from build123d import *

# Parameters (mm, degrees)
SKETCH1_R           = 13
BOSS_EXTRUDE1_DEPTH = 1
CUT_EXTRUDE1_DEPTH  = 1


with BuildPart() as part:
    # Sketch1 → Boss-Extrude1 (new body)
    with BuildSketch(Plane(origin=(0, 0, 0), x_dir=(1, 0, 0), z_dir=(0, 1, 0))):
        with Locations(Location((0, 0, 0), (0, 0, 270))):
            Circle(SKETCH1_R)
    extrude(amount=BOSS_EXTRUDE1_DEPTH)

    # Sketch2 → Cut-Extrude1 (cut)
    with BuildSketch(Plane(origin=(0, 1, 0), x_dir=(1, 0, 0), z_dir=(0, 1, 0))):
        with BuildLine():
            Line((5.25239325, -1.5848325), (7.730691862, -2.231533889))
            add(Edge.make_bspline(
                [(7.730691862, -2.231533889), (7.745854907, -2.465826289), (7.774011213, -2.900884585), (7.780007907, -3.336797312), (7.782775195, -3.5379575)],
                knots=[0, 0, 0, 0, 1.077062099, 2, 2, 2, 2], degree=3))
            add(Edge.make_bspline(
                [(7.782775195, -3.5379575), (7.775734441, -3.772666286), (7.76198387, -4.231051786), (7.665106789, -4.902107863), (7.503534805, -5.53719048), (7.262506376, -6.13254792), (6.970171749, -6.697349561), (6.599918526, -7.220612544), (6.167294917, -7.709069047), (5.673484979, -8.159929958), (5.121589843, -8.561266158), (4.525330961, -8.915315997), (3.88158819, -9.210662332), (3.194771896, -9.454210567), (2.461957382, -9.639228793), (1.685716726, -9.772679799), (0.864809488, -9.857517539), (0.301796476, -9.866054195), (0.013677973, -9.870422778)],
                knots=[0, 0, 0, 0, 0.99838358, 1.9498399, 2.87846334, 3.779167422, 4.676774372, 5.578403417, 6.498521769, 7.448363946, 8.417281084, 9.396931457, 10.393890904, 11.425717394, 12.493153504, 13.605299621, 14.774526564, 16, 16, 16, 16], degree=3))
            add(Edge.make_bspline(
                [(0.013677973, -9.870422778), (-0.345453387, -9.863405493), (-1.042591343, -9.849783693), (-2.054913482, -9.730806098), (-2.997808304, -9.537362324), (-3.874251245, -9.270503592), (-4.678201905, -8.917315993), (-5.411628354, -8.48501399), (-6.080262751, -7.979187866), (-6.671165693, -7.386273411), (-7.201957369, -6.724194549), (-7.653742039, -5.97838427), (-8.036288232, -5.157199578), (-8.347723272, -4.258020447), (-8.589436148, -3.28160554), (-8.760231838, -2.227786178), (-8.865609009, -1.096529571), (-8.877670491, -0.316264728), (-8.883891472, 0.086174444)],
                knots=[0, 0, 0, 0, 1.125976169, 2.185720361, 3.191248848, 4.14129961, 5.053465363, 5.93822711, 6.80577772, 7.675236456, 8.556734678, 9.460955445, 10.40277975, 11.392896532, 12.440517575, 13.553427658, 14.738125192, 16, 16, 16, 16], degree=3))
            add(Edge.make_bspline(
                [(-8.883891472, 0.086174444), (-8.877144448, 0.471355807), (-8.86396985, 1.223481467), (-8.739062258, 2.323761593), (-8.537683843, 3.368297285), (-8.25053484, 4.357501558), (-7.88374945, 5.291207721), (-7.443760547, 6.173716613), (-6.907249974, 6.992501414), (-6.303194776, 7.754037533), (-5.634782916, 8.444869562), (-4.903943631, 9.039841274), (-4.13324793, 9.555570007), (-3.305494781, 9.969042017), (-2.430073405, 10.289949015), (-1.506733392, 10.522051081), (-0.534275431, 10.656589456), (0.130450492, 10.675493327), (0.469407139, 10.685132778)],
                knots=[0, 0, 0, 0, 1.163899941, 2.272693063, 3.342163629, 4.375955692, 5.38130337, 6.37089149, 7.350964679, 8.334427181, 9.30546345, 10.250064938, 11.177916844, 12.10296145, 13.039623816, 13.99100338, 14.975573636, 16, 16, 16, 16], degree=3))
            add(Edge.make_bspline(
                [(0.469407139, 10.685132778), (0.731368093, 10.679403838), (1.24032138, 10.668273314), (1.980031414, 10.603376578), (2.666696134, 10.474000255), (3.305409253, 10.309794879), (3.889173706, 10.08444307), (4.428427211, 9.822804709), (4.914586315, 9.502127233), (5.349181396, 9.133633154), (5.732807037, 8.715102812), (6.062391941, 8.247124839), (6.347469876, 7.733536448), (6.571984508, 7.166341162), (6.748453612, 6.552678606), (6.879804132, 5.890982879), (6.951396325, 5.180354064), (6.961564938, 4.691361745), (6.966802973, 4.439473056)],
                knots=[0, 0, 0, 0, 1.216450272, 2.363391781, 3.442411128, 4.457483076, 5.420551553, 6.342768242, 7.235147886, 8.116718114, 8.981990498, 9.863560726, 10.768467107, 11.70271401, 12.689043052, 13.729727606, 14.830542089, 16, 16, 16, 16], degree=3))
            Line((6.966802973, 4.439473056), (4.475483528, 3.302320278))
            add(Edge.make_bspline(
                [(4.475483528, 3.302320278), (4.470106952, 3.438293944), (4.45992788, 3.695722764), (4.461276647, 4.056170034), (4.447142903, 4.368506474), (4.448715354, 4.55954313), (4.449441862, 4.647806389)],
                knots=[0, 0, 0, 0, 1.21319996, 2.296861169, 3.213111309, 4, 4, 4, 4], degree=3))
            add(Edge.make_bspline(
                [(4.449441862, 4.647806389), (4.447722623, 4.824448026), (4.444391201, 5.166731988), (4.396660933, 5.661731695), (4.337462463, 6.125936258), (4.234766253, 6.552649254), (4.115177918, 6.949061221), (3.964373313, 7.308698933), (3.783801492, 7.63357582), (3.580758496, 7.927608424), (3.344642243, 8.184947546), (3.080877209, 8.407247168), (2.794090455, 8.602656301), (2.472644536, 8.751215907), (2.129602996, 8.876345015), (1.755447324, 8.955010862), (1.356440833, 9.009630083), (1.080143634, 9.015466719), (0.938157139, 9.018466111)],
                knots=[0, 0, 0, 0, 1.322247294, 2.562159472, 3.722092324, 4.823306397, 5.844541812, 6.820517713, 7.73713301, 8.62386865, 9.490450857, 10.343654022, 11.203094787, 12.080246692, 12.988369862, 13.932056947, 14.937303798, 16, 16, 16, 16], degree=3))
            add(Edge.make_bspline(
                [(0.938157139, 9.018466111), (0.786942196, 9.012673682), (0.491913679, 9.001372339), (0.064405318, 8.885963451), (-0.332873883, 8.703985183), (-0.69991465, 8.444701136), (-1.036329743, 8.114914494), (-1.33955244, 7.710706144), (-1.612917553, 7.235906282), (-1.860109833, 6.690970947), (-2.074074797, 6.070923113), (-2.264395958, 5.381001791), (-2.423002996, 4.619720467), (-2.553018757, 3.7867718), (-2.649338988, 2.881263355), (-2.723635136, 1.902892729), (-2.766722621, 0.853348432), (-2.770719009, 0.129616858), (-2.772780361, -0.243686667)],
                knots=[0, 0, 0, 0, 0.663754609, 1.295021072, 1.932796925, 2.5771421, 3.261147111, 3.996780335, 4.792416042, 5.666644777, 6.624635675, 7.674451774, 8.812674813, 10.04299616, 11.380987675, 12.816846398, 14.358117152, 16, 16, 16, 16], degree=3))
            add(Edge.make_bspline(
                [(-2.772780361, -0.243686667), (-2.769234908, -0.564921798), (-2.762363487, -1.187505667), (-2.715752199, -2.089773852), (-2.634330422, -2.929957842), (-2.518780135, -3.708339901), (-2.367195765, -4.425682347), (-2.18616641, -5.08138104), (-1.977536957, -5.676945191), (-1.721955983, -6.20495828), (-1.442920917, -6.676002474), (-1.128010362, -7.08687999), (-0.775787049, -7.432245929), (-0.387635905, -7.711578053), (0.02746432, -7.94149635), (0.483873953, -8.086328054), (0.968240334, -8.189856946), (1.303586281, -8.199030191), (1.476351584, -8.203756111)],
                knots=[0, 0, 0, 0, 1.528653098, 2.962673341, 4.297845131, 5.544148307, 6.705400685, 7.784456391, 8.779695543, 9.703504234, 10.571332445, 11.381068858, 12.160045423, 12.90918257, 13.651518771, 14.406987965, 15.179303616, 16, 16, 16, 16], degree=3))
            add(Edge.make_bspline(
                [(1.476351584, -8.203756111), (1.61974551, -8.199179957), (1.902048757, -8.190170766), (2.316640973, -8.13115633), (2.709880212, -8.019466978), (3.085346323, -7.871676439), (3.444251194, -7.683979914), (3.784176044, -7.453188362), (4.102744826, -7.17621313), (4.399160241, -6.860901751), (4.671310822, -6.515633609), (4.911973057, -6.146309401), (5.111323132, -5.752451865), (5.277229417, -5.340485015), (5.402928553, -4.906821297), (5.493239479, -4.453833285), (5.552273744, -3.979325579), (5.557758131, -3.655325036), (5.560552973, -3.490214444)],
                knots=[0, 0, 0, 0, 0.988561849, 1.946206698, 2.877739568, 3.799990945, 4.723373952, 5.6638324, 6.625467346, 7.627221263, 8.642730559, 9.652395785, 10.660385053, 11.680779451, 12.709570302, 13.767670509, 14.862405475, 16, 16, 16, 16], degree=3))
            add(Edge.make_bspline(
                [(5.560552973, -3.490214444), (5.557098155, -3.369930029), (5.549404006, -3.102047251), (5.479283066, -2.663994986), (5.38676253, -2.147904033), (5.299251417, -1.781190622), (5.25239325, -1.5848325)],
                knots=[0, 0, 0, 0, 0.745982987, 1.661362321, 2.747767356, 4, 4, 4, 4], degree=3))
        make_face()
    extrude(amount=-CUT_EXTRUDE1_DEPTH, mode=Mode.SUBTRACT)


solid = part.part
Verification items for the finished model (mm, model axes). A direction names the side the tool comes from. Coordinates: 2 decimals unless noted, no trailing zeros. Order: outer loops, then holes, each group sorted by start corner. A loop starts at its lowest first (then second) coordinate and runs counter-clockwise, first axis right, second up. Notation, with made-up numbers: (81, -23) -> (126, -23) arc R25 ccw to (126, 5) -> close; hole circle Ø4 at (-29, -20). An arc over 180 degrees is marked (long way). Put each result on its own line as item: value. Start each with the question number.
1. Material ranges on L1, parallel to X at y = 0.15, z = -4.25; L2, parallel to Z at x = 3, y = 0.15; L3, parallel to X at y = 0.25, z = -6.75, recorded low to high. Write a range as [from, to].
2. Access from +Z, -Z, +X, -X, +Y, -Y to the whole of each face (thin tool, end or side, straight path). Record for faces 1 (the flat face through (5.74, 0.51, -3.88)), 2 (the flat face through (0, 0, 0)).
3. Cross-section at A-A, the plane z = 4. Count the separate pieces of the cut face and the enclosed holes in it, then the cut area to 3 significant figures.
4. Mould release check, pull along Z, two halves, no side actions. Record for faces 3 (the flat face through (6.474, 0.507, 1.904)), 4 (the cylindrical face through (-7.91, 0.493, -10.316)), 5 (the flat face through (0, 1, 0)): released by +Z, released by -Z, zero draft, split by the parting line, or undercut.
5. Cross-section at B-B, the plane x = 10. Record the boundary of the cut face in (y, z), then the cut area to 3 significant figures.
Computed:
1. L1: [-12.29, -8.27], [-2.48, 4.45], [6.55, 12.29]
1. L2: [-12.65, -10.39], [-8.46, 7.9], [9.5, 12.65]
1. L3: [-11.11, -7.06], [-1.83, 4.17], [6.69, 11.11]
2. face 1: +Y, -Y
2. face 2: +Z, -Z, +X, -X, -Y
3. separate pieces: 3
3. enclosed holes: 0
3. area: 16.6 mm2
4. face 3: undercut
4. face 4: split by the parting line
4. face 5: zero draft
5. outline: (0, -8.31) -> (1, -8.31) -> (1, 8.31) -> (0, 8.31) -> close
5. area: 16.6 mm2
